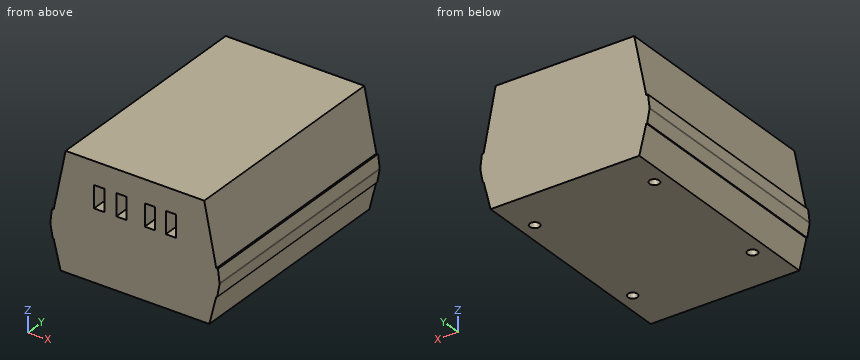
from build123d import *

# Parameters (mm, degrees)
F0_W     = 98.933
F0_H     = 132.2578
F1_DEPTH = 67.31
F3_DEPTH = 132.2578
F4_W     = 5.994986
F4_H     = 12.929627
F5_DEPTH = 12.7
F6_R     = 2.8575
F7_DEPTH = 9.144


with BuildPart() as f1:
    # F0 (on Top) → F1 (new body)
    with BuildSketch(Plane.XY):
        Rectangle(F0_W, F0_H)
    extrude(amount=F1_DEPTH)

    # F2 (on face) → F3 (cut, through all)
    with BuildSketch(Plane.XZ.offset(66.1289)):
        Polygon((-47.556915, 32.258), (-40.523797, 67.31), (-49.4665, 67.31), (-49.4665, 24.638), (-48.539754, 32.258), align=None)
        Polygon((-48.057587, 16.51), (-49.4665, 24.055742), (-49.4665, 0), (-43.474339, 0), (-47.556915, 16.51), align=None)
        Polygon((49.4665, 0), (49.4665, 24.055742), (48.057587, 16.51), (47.556915, 16.51), (43.474339, 0), align=None)
        Polygon((49.4665, 67.31), (40.523797, 67.31), (47.556915, 32.258), (48.539754, 32.258), (49.4665, 24.638), align=None)
    extrude(amount=-F3_DEPTH, mode=Mode.SUBTRACT)

    # F4 (on face) → F5 (cut)
    with BuildSketch(Plane.XZ.offset(66.1289)):
        with Locations((-20.924805, 47.556382)):
            Rectangle(F4_W, F4_H)
        with Locations((-7.897241, 47.556382)):
            Rectangle(F4_W, F4_H)
        with Locations((8.76972, 47.556382)):
            Rectangle(F4_W, F4_H)
        with Locations((21.055504, 47.556382)):
            Rectangle(F4_W, F4_H)
    extrude(amount=-F5_DEPTH, mode=Mode.SUBTRACT)

    # F6 (on face) → F7 (cut)
    with BuildSketch(Plane(origin=(0, 0, 0), x_dir=(1, 0, 0), z_dir=(0, 0, -1))):
        with Locations((-35.0012, -41.6814)):
            Circle(F6_R)
        with Locations((35.0012, -41.6814)):
            Circle(F6_R)
        with Locations((35.0012, 39.3192)):
            Circle(F6_R)
        with Locations((-35.0012, 39.3192)):
            Circle(F6_R)
    extrude(amount=-F7_DEPTH, mode=Mode.SUBTRACT)


solid = f1.part
Build history of the part. All positions in model axes, mm. Coordinates: 2 decimals unless noted, no trailing zeros. Order: outer loops, then holes, each group sorted by start corner. A loop starts at its lowest first (then second) coordinate and runs counter-clockwise, first axis right, second up. Notation, with made-up numbers: (69.25, -39) - (113.25, -39) arc R35 ccw to (113.25, -7) - close; hole circle Ø5 at (70, 20). An arc over 180 degrees is marked (long way). Put each result on its own line as item: value.
1. Drop flat-ended pins along their axis: P1, Ø4, axis at y = -60, z = 45.5, coming from the +X side; P2, Ø4, axis at y = -57.5, z = 46, coming from the +X side; P3, Ø4.5, axis at x = 35, y = 43, coming from the -Z side; P4, Ø1, axis at y = -26, z = 60, coming from the +X side. Give the stop position or say it passes through.
Answer sheet:
P1: stops at x = 45.3
P2: stops at x = 45.2
P3: stops at z = 0
P4: stops at x = 42.09
2. Saw through at D-D (z = 18). Write the cut outline in (x, y).
Answer sheet:
outline: (-48.34, -66.13) - (48.34, -66.13) - (48.34, 66.13) - (-48.34, 66.13) - close
3. Saw through at C-C (z = 47.5). Write the cut outline in (x, y), and give its area (3 significant figures).
Answer sheet:
outline: (-44.5, -66.13) - (-23.92, -66.13) - (-23.92, -53.43) - (-17.93, -53.43) - (-17.93, -66.13) - (-10.89, -66.13) - (-10.89, -53.43) - (-4.9, -53.43) - (-4.9, -66.13) - (5.77, -66.13) - (5.77, -53.43) - (11.77, -53.43) - (11.77, -66.13) - (18.06, -66.13) - (18.06, -53.43) - (24.05, -53.43) - (24.05, -66.13) - (44.5, -66.13) - (44.5, 66.13) - (-44.5, 66.13) - close
area: 11,500 mm^2
4. Probe line 1 along X through (y, z) = (39.5, 24); line 2 along X through (y, z) = (2, 61.5). List the from-to ranges inside material, lowest first. Write a range as [from, to].
Answer sheet:
line 1: x = [-49.46, 49.46]
line 2: x = [-41.69, 41.69]
5. Saw through at A-A (x = 20). Write the cut outline in (y, z), and give its area (3 significant figures).
Answer sheet:
outline: (-66.13, 0) - (66.13, 0) - (66.13, 67.31) - (-66.13, 67.31) - (-66.13, 54.02) - (-53.43, 54.02) - (-53.43, 41.09) - (-66.13, 41.09) - close
area: 8,740 mm^2
6. Saw through at B-B (y = 28.5). Write the cut outline in (x, z), and give its area (3 significant figures).
Answer sheet:
outline: (-49.47, 24.06) - (-48.06, 16.51) - (-47.56, 16.51) - (-43.47, 0) - (43.47, 0) - (47.56, 16.51) - (48.06, 16.51) - (49.47, 24.06) - (49.47, 24.64) - (48.54, 32.26) - (47.56, 32.26) - (40.52, 67.31) - (-40.52, 67.31) - (-47.56, 32.26) - (-48.54, 32.26) - (-49.47, 24.64) - close
area: 6,130 mm^2
